The model under review builds one solid part; all positions refer to its coordinate system, in mm. Face numbers are marked on the shaded views. A direction names the side the tool comes from. Coordinates: 2 decimals unless noted, no trailing zeros. Order: outer loops, then holes, each group sorted by start corner. A loop starts at its lowest first (then second) coordinate and runs counter-clockwise, first axis right, second up.
from build123d import *

# Parameters (mm, degrees)
SKETCH1_R                 = 12.5
BOSS_EXTRUDE1_DEPTH       = 60
SKETCH2_R                 = 3.5
BOSS_EXTRUDE2_DEPTH       = 2.5
SKETCH2_3_R               = 2
BOSS_EXTRUDE3_DEPTH       = 12
M3X0_5_TAPPED_HOLE1_D     = 2.5
M3X0_5_TAPPED_HOLE1_DEPTH = 4.99999
M3X0_5_TAPPED_HOLE1_TIP   = 0.751075774
CUT_EXTRUDE1_START        = -0.5
SKETCH6_R                 = 12.5
SKETCH6_R_2               = 12.2
CUT_EXTRUDE1_DEPTH        = 0.5
SKETCH5_R                 = 7
BOSS_EXTRUDE4_DEPTH       = 9


with BuildPart() as part:
    # Sketch1 → Boss-Extrude1 (new body)
    with BuildSketch(Plane.XY):
        Circle(SKETCH1_R)
    extrude(amount=-BOSS_EXTRUDE1_DEPTH)

    # Sketch2 → Boss-Extrude2 (add)
    with BuildSketch(Plane.XY):
        Circle(SKETCH2_R)
    extrude(amount=BOSS_EXTRUDE2_DEPTH)

    # Sketch2_3 → Boss-Extrude3 (add)
    with BuildSketch(Plane.XY):
        Circle(SKETCH2_3_R)
    extrude(amount=BOSS_EXTRUDE3_DEPTH)

    # M3x0.5 Tapped Hole1
    with Locations(Plane.XY):
        with Locations((0, 8.5), (0, -8.5)):
            Hole(M3X0_5_TAPPED_HOLE1_D / 2, depth=M3X0_5_TAPPED_HOLE1_DEPTH)
            with Locations((0, 0, -(M3X0_5_TAPPED_HOLE1_DEPTH + M3X0_5_TAPPED_HOLE1_TIP / 2))):  # 118° drill point
                Cone(0, M3X0_5_TAPPED_HOLE1_D / 2, M3X0_5_TAPPED_HOLE1_TIP, mode=Mode.SUBTRACT)

    # Sketch6 → Cut-Extrude1 (cut)
    with BuildSketch(Plane(origin=(0, 0, -60), x_dir=(-1, 0, 0), z_dir=(0, 0, -1)).offset(CUT_EXTRUDE1_START)):
        with Locations(Location((0, 0, 0), (0, 0, 180))):
            Circle(SKETCH6_R)
        Circle(SKETCH6_R_2, mode=Mode.SUBTRACT)
    extrude(amount=CUT_EXTRUDE1_DEPTH, mode=Mode.SUBTRACT)

    # Sketch5 → Boss-Extrude4 (add)
    with BuildSketch(Plane(origin=(0, 0, -60), x_dir=(-1, 0, 0), z_dir=(0, 0, -1))):
        Circle(SKETCH5_R)
    extrude(amount=BOSS_EXTRUDE4_DEPTH)


solid = part.part
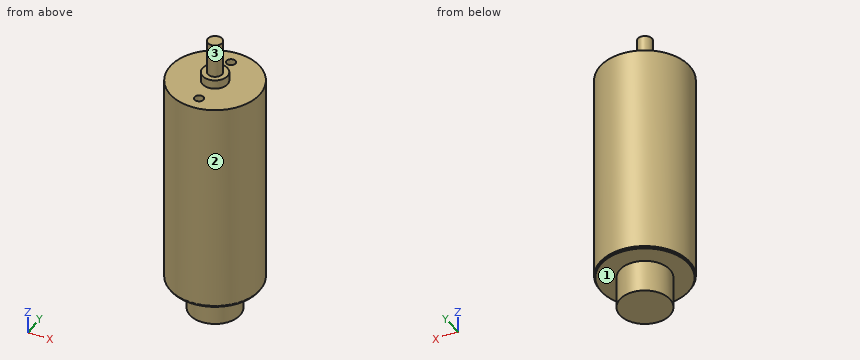
(1) Tool access review of the marked faces 1, 2 and 3: name each direction out of +Z, -Z, +X, -X, +Y, -Y from which nothing blocks a thin tool from reaching the whole face with its end or side.
(2) Consider section C-C (x = -9.75). Give the boundary of the cut face in (y, z).
(3) Consider section B-B (z = -30.5). Give the boundary of the cut face in (x, y).
(4) Consider section A-A (y = 0). Give the boundary of the cut face in (x, z), then the cut area to 3 significant figures.
(5) Wall thickness on line 1 (Y direction, x = 0, z = -2.2); line 2 (Z direction, x = -3.25, y = -0.5); line 3 (Z direction, x = -2.5, y = 5.75): over which ranges is each line inside the solid? List them lowest first.
(6) Consider section D-D (z = -1.5). Give the boundary of the cut face in (x, y).
(7) Insertion check: pin 1 Ø8 at (x, z) = (-5, 2.5) entering from +Y; pin 2 Ø10 at (y, z) = (2.5, -50.5) entering from +X; pin 3 Ø6 at (x, y) = (5.5, 0.5) entering from +Z; pin 4 Ø1.5 at (y, z) = (-4, -21) entering from +X. Each pin has a flat end and moves straight along its axis. Give the tip position at first contact, or say it passes through.
Findings:
1. face 1: -Z
1. face 2: +Z, -Z
1. face 3: +Z
2. outline: (-7.82, -59.5) - (-7.33, -59.5) - (-7.33, -60) - (7.33, -60) - (7.33, -59.5) - (7.82, -59.5) - (7.82, 0) - (-7.82, 0) - close
3. outline: circle Ø25 at (0, 0)
4. outline: (-12.5, -59.5) - (-12.2, -59.5) - (-12.2, -60) - (-7, -60) - (-7, -69) - (7, -69) - (7, -60) - (12.2, -60) - (12.2, -59.5) - (12.5, -59.5) - (12.5, 0) - (3.5, 0) - (3.5, 2.5) - (2, 2.5) - (2, 12) - (-2, 12) - (-2, 2.5) - (-3.5, 2.5) - (-3.5, 0) - (-12.5, 0) - close
4. area: 1,680 mm2
5. line 1: y = -12.5 to -9.75, -7.25 to 7.25, 9.75 to 12.5
5. line 2: z = -69 to 2.5
5. line 3: z = -69 to 0
6. outline: circle Ø25 at (0, 0); hole circle Ø2.5 at (0, -8.5); hole circle Ø2.5 at (0, 8.5)
7. pin 1: stops at y = 12.36
7. pin 2: stops at x = 12.5
7. pin 3: stops at z = 2.5
7. pin 4: stops at x = 12.07
